Can you work these out from the model? Positions are in its coordinate system, mm. Face numbers are marked on the shaded views. A direction names the side the tool comes from. Coordinates: 2 decimals unless noted, no trailing zeros. Order: outer loops, then holes, each group sorted by start corner. A loop starts at its lowest first (then second) coordinate and runs counter-clockwise, first axis right, second up. Notation, with made-up numbers: (-26, -18.75) -> (11, -18.75) arc R12 ccw to (11, -4.75) -> close; hole circle Ø11 at (75.5, 80.25). An arc over 180 degrees is marked (long way). Answer in a Markdown table with one row per item.
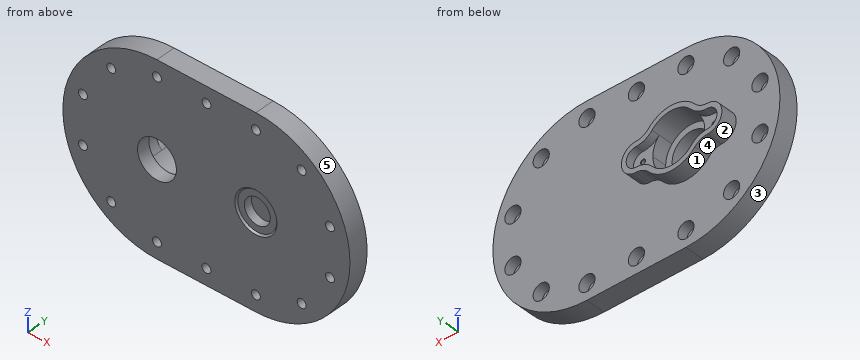
```python
from build123d import *

# Parameters (mm, degrees)
SKETCH2_R                   = 5
BOSS_EXTRUDE4_DEPTH         = 12
SKETCH2_6_R                 = 16
SKETCH2_6_R_2               = 12
BOSS_EXTRUDE5_DEPTH         = 8
SKETCH2_7_R                 = 1.25
BOSS_EXTRUDE6_DEPTH         = 17
BOSS_EXTRUDE7_DEPTH         = 22
SKETCH2_10_R                = 1.25
BOSS_EXTRUDE9_DEPTH         = 17
M3_TAPPED_HOLE2_D           = 2.5
M3_TAPPED_HOLE2_DEPTH       = 10
M3_TAPPED_HOLE2_CSINK_D     = 3.05
M3_TAPPED_HOLE2_CSINK_ANGLE = 90
M3_TAPPED_HOLE2_TIP         = 0.751075774
SKETCH11_R                  = 12
CUT_EXTRUDE1_DEPTH          = 1
SKETCH12_R                  = 8
CUT_EXTRUDE2_DEPTH          = 6
CHAMFER1_SIZE               = 1
SKETCH2_12_R                = 5
SKETCH2_12_R_2              = 2.75
BOSS_EXTRUDE10_DEPTH        = 5.8


with BuildPart() as part:
    # Sketch2 → Boss-Extrude4 (new body)
    with BuildSketch(Plane(origin=(0, 0, 0), x_dir=(1, 0, 0), z_dir=(0, 1, 0))):
        with BuildLine():
            Line((-61, -58), (0, -58))
            ThreePointArc((0, -58), (58, 0), (0, 58))
            Line((0, 58), (-61, 58))
            ThreePointArc((-61, 58), (-119, 0), (-61, -58))
        make_face()
        with Locations(Location((0, 48, 0), (0, 0, 270))):
            Circle(SKETCH2_R, mode=Mode.SUBTRACT)
        with Locations(Location((-30.5, 48, 0), (0, 0, 270))):
            Circle(SKETCH2_R, mode=Mode.SUBTRACT)
        with Locations(Location((-61, 48, 0), (0, 0, 270))):
            Circle(SKETCH2_R, mode=Mode.SUBTRACT)
        with Locations(Location((-89.21369211, 38.83281573, 0), (0, 0, 270))):
            Circle(SKETCH2_R, mode=Mode.SUBTRACT)
        with Locations(Location((-106.650712782, 14.83281573, 0), (0, 0, 270))):
            Circle(SKETCH2_R, mode=Mode.SUBTRACT)
        with Locations(Location((-106.650712782, -14.83281573, 0), (0, 0, 270))):
            Circle(SKETCH2_R, mode=Mode.SUBTRACT)
        with Locations(Location((-89.21369211, -38.83281573, 0), (0, 0, 270))):
            Circle(SKETCH2_R, mode=Mode.SUBTRACT)
        with Locations(Location((-61, -48, 0), (0, 0, 270))):
            Circle(SKETCH2_R, mode=Mode.SUBTRACT)
        with Locations(Location((-30.5, -48, 0), (0, 0, 270))):
            Circle(SKETCH2_R, mode=Mode.SUBTRACT)
        with Locations(Location((0, -48, 0), (0, 0, 270))):
            Circle(SKETCH2_R, mode=Mode.SUBTRACT)
        with Locations(Location((28.21369211, -38.83281573, 0), (0, 0, 270))):
            Circle(SKETCH2_R, mode=Mode.SUBTRACT)
        with Locations(Location((45.650712782, -14.83281573, 0), (0, 0, 270))):
            Circle(SKETCH2_R, mode=Mode.SUBTRACT)
        with Locations(Location((45.650712782, 14.83281573, 0), (0, 0, 270))):
            Circle(SKETCH2_R, mode=Mode.SUBTRACT)
        with Locations(Location((28.21369211, 38.83281573, 0), (0, 0, 270))):
            Circle(SKETCH2_R, mode=Mode.SUBTRACT)
        with BuildLine():
            ThreePointArc((-75.315068493, -12.493150685), (-61, -19), (-46.684931507, -12.493150685))
            ThreePointArc((-46.684931507, -12.493150685), (-43.220790032, -9.91426193), (-39, -9))
            ThreePointArc((-39, -9), (-30, 0), (-39, 9))
            ThreePointArc((-39, 9), (-43.220790032, 9.91426193), (-46.684931507, 12.493150685))
            ThreePointArc((-46.684931507, 12.493150685), (-61, 19), (-75.315068493, 12.493150685))
            ThreePointArc((-75.315068493, 12.493150685), (-78.779209968, 9.91426193), (-83, 9))
            ThreePointArc((-83, 9), (-92, 0), (-83, -9))
            ThreePointArc((-83, -9), (-78.779209968, -9.91426193), (-75.315068493, -12.493150685))
        make_face(mode=Mode.SUBTRACT)
    extrude(amount=BOSS_EXTRUDE4_DEPTH)



with BuildPart() as body_2:
    # Sketch2<6> → Boss-Extrude5 (new body)
    with BuildSketch(Plane(origin=(0, 0, 0), x_dir=(1, 0, 0), z_dir=(0, 1, 0))):
        with Locations(Location((-61, 0, 0), (0, 0, 270))):
            Circle(SKETCH2_6_R)
        with Locations(Location((-61, 0, 0), (0, 0, 270))):
            Circle(SKETCH2_6_R_2, mode=Mode.SUBTRACT)
    extrude(amount=BOSS_EXTRUDE5_DEPTH)

    # Sketch2<7> → Boss-Extrude6 (add)
    # profile 1 of 2: a face of its own
    with BuildSketch(Plane(origin=(0, 0, 0), x_dir=(1, 0, 0), z_dir=(0, 1, 0))):
        with BuildLine():
            ThreePointArc((-48.945205479, 10.520547945), (-46.018733159, 5.617975065), (-45, 0))
            ThreePointArc((-45, 0), (-46.018733159, -5.617975065), (-48.945205479, -10.520547945))
            ThreePointArc((-48.945205479, -10.520547945), (-44.462198865, -7.183162497), (-39, -6))
            ThreePointArc((-39, -6), (-33, 0), (-39, 6))
            ThreePointArc((-39, 6), (-44.462198865, 7.183162497), (-48.945205479, 10.520547945))
        make_face()
        with Locations(Location((-39, 0, 0), (0, 0, 270))):
            Circle(SKETCH2_7_R, mode=Mode.SUBTRACT)
    # profile 2 of 2: a face of its own
    with BuildSketch(Plane(origin=(0, 0, 0), x_dir=(1, 0, 0), z_dir=(0, 1, 0))):
        with BuildLine():
            ThreePointArc((-73.054794521, -10.520547945), (-77, 0), (-73.054794521, 10.520547945))
            ThreePointArc((-73.054794521, 10.520547945), (-77.537801135, 7.183162497), (-83, 6))
            ThreePointArc((-83, 6), (-89, 0), (-83, -6))
            ThreePointArc((-83, -6), (-77.537801135, -7.183162497), (-73.054794521, -10.520547945))
        make_face()
        with Locations(Location((-83, 0, 0), (0, 0, 270))):
            Circle(SKETCH2_7_R, mode=Mode.SUBTRACT)
    extrude(amount=BOSS_EXTRUDE6_DEPTH)


with BuildPart() as part_1:
    add(part.part)

    add(body_2.part)  # Boss-Extrude7 merges body 2
    # Sketch2<8> → Boss-Extrude7 (add)
    with BuildSketch(Plane(origin=(0, 0, 0), x_dir=(1, 0, 0), z_dir=(0, 1, 0))):
        with BuildLine():
            ThreePointArc((-46.684931507, -12.493150685), (-43.220790032, -9.91426193), (-39, -9))
            ThreePointArc((-39, -9), (-30, 0), (-39, 9))
            ThreePointArc((-39, 9), (-43.220790032, 9.91426193), (-46.684931507, 12.493150685))
            ThreePointArc((-46.684931507, 12.493150685), (-61, 19), (-75.315068493, 12.493150685))
            ThreePointArc((-75.315068493, 12.493150685), (-78.779209968, 9.91426193), (-83, 9))
            ThreePointArc((-83, 9), (-92, 0), (-83, -9))
            ThreePointArc((-83, -9), (-78.779209968, -9.91426193), (-75.315068493, -12.493150685))
            ThreePointArc((-75.315068493, -12.493150685), (-61, -19), (-46.684931507, -12.493150685))
        make_face()
        with BuildLine():
            ThreePointArc((-48.945205479, 10.520547945), (-44.462198865, 7.183162497), (-39, 6))
            ThreePointArc((-39, 6), (-33, 0), (-39, -6))
            ThreePointArc((-39, -6), (-44.462198865, -7.183162497), (-48.945205479, -10.520547945))
            ThreePointArc((-48.945205479, -10.520547945), (-61, -16), (-73.054794521, -10.520547945))
            ThreePointArc((-73.054794521, -10.520547945), (-77.537801135, -7.183162497), (-83, -6))
            ThreePointArc((-83, -6), (-89, 0), (-83, 6))
            ThreePointArc((-83, 6), (-77.537801135, 7.183162497), (-73.054794521, 10.520547945))
            ThreePointArc((-73.054794521, 10.520547945), (-61, 16), (-48.945205479, 10.520547945))
        make_face(mode=Mode.SUBTRACT)
    extrude(amount=BOSS_EXTRUDE7_DEPTH)

    # Sketch2<10> → Boss-Extrude9 (add)
    with BuildSketch(Plane(origin=(0, 0, 0), x_dir=(1, 0, 0), z_dir=(0, 1, 0))):
        with Locations((-39, 0)):
            Circle(SKETCH2_10_R)
        with Locations((-83, 0)):
            Circle(SKETCH2_10_R)
    extrude(amount=BOSS_EXTRUDE9_DEPTH)

    # M3 Tapped Hole2
    with Locations(Plane(origin=(0, 17, 0), x_dir=(1, 0, 0), z_dir=(0, 1, 0))):
        with Locations((-39, 0), (-83, 0)):
            CounterSinkHole(M3_TAPPED_HOLE2_D / 2, M3_TAPPED_HOLE2_CSINK_D / 2, depth=M3_TAPPED_HOLE2_DEPTH, counter_sink_angle=M3_TAPPED_HOLE2_CSINK_ANGLE)
            with Locations((0, 0, -(M3_TAPPED_HOLE2_DEPTH + M3_TAPPED_HOLE2_TIP / 2))):  # 118° drill point
                Cone(0, M3_TAPPED_HOLE2_D / 2, M3_TAPPED_HOLE2_TIP, mode=Mode.SUBTRACT)

    # Sketch11 → Cut-Extrude1 (cut)
    with BuildSketch(Plane.XZ):
        with Locations(Location((0, 0, 0), (0, 0, 270))):
            Circle(SKETCH11_R)
    extrude(amount=-CUT_EXTRUDE1_DEPTH, mode=Mode.SUBTRACT)

    # Sketch12 → Cut-Extrude2 (cut)
    with BuildSketch(Plane.XZ):
        with Locations(Location((0, 0, 0), (0, 0, 270))):
            Circle(SKETCH12_R)
    extrude(amount=-CUT_EXTRUDE2_DEPTH, mode=Mode.SUBTRACT)

    # Chamfer1
    chamfer1_edges = [part_1.edges().sort_by_distance(p)[0] for p in [
        (0, 0, 12),
    ]]
    chamfer(chamfer1_edges, length=CHAMFER1_SIZE - 0.0001)  # a hair under: the kernel refuses the full size

    # Sketch2<12> → Boss-Extrude10 (add)
    # profile 1 of 14: a face of its own
    with BuildSketch(Plane(origin=(0, 0, 0), x_dir=(1, 0, 0), z_dir=(0, 1, 0))):
        with Locations(Location((0, -48, 0), (0, 0, 270))):
            Circle(SKETCH2_12_R)
        with Locations(Location((0, -48, 0), (0, 0, 270))):
            Circle(SKETCH2_12_R_2, mode=Mode.SUBTRACT)
    # profile 2 of 14: a face of its own
    with BuildSketch(Plane(origin=(0, 0, 0), x_dir=(1, 0, 0), z_dir=(0, 1, 0))):
        with Locations(Location((28.21369211, -38.83281573, 0), (0, 0, 270))):
            Circle(SKETCH2_12_R)
        with Locations(Location((28.21369211, -38.83281573, 0), (0, 0, 270))):
            Circle(SKETCH2_12_R_2, mode=Mode.SUBTRACT)
    # profile 3 of 14: a face of its own
    with BuildSketch(Plane(origin=(0, 0, 0), x_dir=(1, 0, 0), z_dir=(0, 1, 0))):
        with Locations(Location((45.650712782, -14.83281573, 0), (0, 0, 270))):
            Circle(SKETCH2_12_R)
        with Locations(Location((45.650712782, -14.83281573, 0), (0, 0, 270))):
            Circle(SKETCH2_12_R_2, mode=Mode.SUBTRACT)
    # profile 4 of 14: a face of its own
    with BuildSketch(Plane(origin=(0, 0, 0), x_dir=(1, 0, 0), z_dir=(0, 1, 0))):
        with Locations(Location((45.650712782, 14.83281573, 0), (0, 0, 270))):
            Circle(SKETCH2_12_R)
        with Locations(Location((45.650712782, 14.83281573, 0), (0, 0, 270))):
            Circle(SKETCH2_12_R_2, mode=Mode.SUBTRACT)
    # profile 5 of 14: a face of its own
    with BuildSketch(Plane(origin=(0, 0, 0), x_dir=(1, 0, 0), z_dir=(0, 1, 0))):
        with Locations(Location((28.21369211, 38.83281573, 0), (0, 0, 270))):
            Circle(SKETCH2_12_R)
        with Locations(Location((28.21369211, 38.83281573, 0), (0, 0, 270))):
            Circle(SKETCH2_12_R_2, mode=Mode.SUBTRACT)
    # profile 6 of 14: a face of its own
    with BuildSketch(Plane(origin=(0, 0, 0), x_dir=(1, 0, 0), z_dir=(0, 1, 0))):
        with Locations(Location((0, 48, 0), (0, 0, 270))):
            Circle(SKETCH2_12_R)
        with Locations(Location((0, 48, 0), (0, 0, 270))):
            Circle(SKETCH2_12_R_2, mode=Mode.SUBTRACT)
    # profile 7 of 14: a face of its own
    with BuildSketch(Plane(origin=(0, 0, 0), x_dir=(1, 0, 0), z_dir=(0, 1, 0))):
        with Locations(Location((-30.5, 48, 0), (0, 0, 270))):
            Circle(SKETCH2_12_R)
        with Locations(Location((-30.5, 48, 0), (0, 0, 270))):
            Circle(SKETCH2_12_R_2, mode=Mode.SUBTRACT)
    # profile 8 of 14: a face of its own
    with BuildSketch(Plane(origin=(0, 0, 0), x_dir=(1, 0, 0), z_dir=(0, 1, 0))):
        with Locations(Location((-61, 48, 0), (0, 0, 270))):
            Circle(SKETCH2_12_R)
        with Locations(Location((-61, 48, 0), (0, 0, 270))):
            Circle(SKETCH2_12_R_2, mode=Mode.SUBTRACT)
    # profile 9 of 14: a face of its own
    with BuildSketch(Plane(origin=(0, 0, 0), x_dir=(1, 0, 0), z_dir=(0, 1, 0))):
        with Locations(Location((-89.21369211, 38.83281573, 0), (0, 0, 270))):
            Circle(SKETCH2_12_R)
        with Locations(Location((-89.21369211, 38.83281573, 0), (0, 0, 270))):
            Circle(SKETCH2_12_R_2, mode=Mode.SUBTRACT)
    # profile 10 of 14: a face of its own
    with BuildSketch(Plane(origin=(0, 0, 0), x_dir=(1, 0, 0), z_dir=(0, 1, 0))):
        with Locations(Location((-106.650712782, 14.83281573, 0), (0, 0, 270))):
            Circle(SKETCH2_12_R)
        with Locations(Location((-106.650712782, 14.83281573, 0), (0, 0, 270))):
            Circle(SKETCH2_12_R_2, mode=Mode.SUBTRACT)
    # profile 11 of 14: a face of its own
    with BuildSketch(Plane(origin=(0, 0, 0), x_dir=(1, 0, 0), z_dir=(0, 1, 0))):
        with Locations(Location((-106.650712782, -14.83281573, 0), (0, 0, 270))):
            Circle(SKETCH2_12_R)
        with Locations(Location((-106.650712782, -14.83281573, 0), (0, 0, 270))):
            Circle(SKETCH2_12_R_2, mode=Mode.SUBTRACT)
    # profile 12 of 14: a face of its own
    with BuildSketch(Plane(origin=(0, 0, 0), x_dir=(1, 0, 0), z_dir=(0, 1, 0))):
        with Locations(Location((-89.21369211, -38.83281573, 0), (0, 0, 270))):
            Circle(SKETCH2_12_R)
        with Locations(Location((-89.21369211, -38.83281573, 0), (0, 0, 270))):
            Circle(SKETCH2_12_R_2, mode=Mode.SUBTRACT)
    # profile 13 of 14: a face of its own
    with BuildSketch(Plane(origin=(0, 0, 0), x_dir=(1, 0, 0), z_dir=(0, 1, 0))):
        with Locations(Location((-61, -48, 0), (0, 0, 270))):
            Circle(SKETCH2_12_R)
        with Locations(Location((-61, -48, 0), (0, 0, 270))):
            Circle(SKETCH2_12_R_2, mode=Mode.SUBTRACT)
    # profile 14 of 14: a face of its own
    with BuildSketch(Plane(origin=(0, 0, 0), x_dir=(1, 0, 0), z_dir=(0, 1, 0))):
        with Locations(Location((-30.5, -48, 0), (0, 0, 270))):
            Circle(SKETCH2_12_R)
        with Locations(Location((-30.5, -48, 0), (0, 0, 270))):
            Circle(SKETCH2_12_R_2, mode=Mode.SUBTRACT)
    extrude(amount=BOSS_EXTRUDE10_DEPTH)


solid = part_1.part
```
(1) Suppose I cut it at C-C (z = -48). Please give me the cut outline in (x, y).
Response values:
| item | result |
|---|---|
| outline | (-93.56, 0) -> (-63.75, 0) -> (-63.75, 5.8) -> (-66, 5.8) -> (-66, 12) -> (-93.56, 12) -> close; (-58.25, 0) -> (-33.25, 0) -> (-33.25, 5.8) -> (-35.5, 5.8) -> (-35.5, 12) -> (-56, 12) -> (-56, 5.8) -> (-58.25, 5.8) -> close; (-27.75, 0) -> (-2.75, 0) -> (-2.75, 5.8) -> (-5, 5.8) -> (-5, 12) -> (-25.5, 12) -> (-25.5, 5.8) -> (-27.75, 5.8) -> close; (2.75, 0) -> (32.56, 0) -> (32.56, 12) -> (5, 12) -> (5, 5.8) -> (2.75, 5.8) -> close |
(2) Suppose I cut it at B-B (x = -52). Please give me the cut outline in (y, z).
Response values:
| item | result |
|---|---|
| outline | (0, -58) -> (12, -58) -> (12, -16.73) -> (22, -16.73) -> (22, -13.23) -> (8, -13.23) -> (8, -7.94) -> (0, -7.94) -> close; (0, 7.94) -> (8, 7.94) -> (8, 13.23) -> (22, 13.23) -> (22, 16.73) -> (12, 16.73) -> (12, 58) -> (0, 58) -> close |
(3) Suppose I cut it at D-D (y = 3.25). Count the separate pieces of the cut face and the enclosed holes in it, and give its area (3 significant figures).
Response values:
| item | result |
|---|---|
| separate pieces | 1 |
| enclosed holes | 16 |
| area | 16,700 mm2 |
(4) On a 3-axis mill with a long thin cutter (end or side, diameter ignored), from which of +Z, -Z, +X, -X, +Y, -Y can I reach the whole of each face in a straight line? I mean the marked faces 1, 2, 3, 4 and 5. Say none if no direction works.
Response values:
| item | result |
|---|---|
| face 1 | -Z, +Y |
| face 2 | -X, +Y |
| face 3 | -X, +Y, -Y |
| face 4 | -Z, -X, +Y |
| face 5 | +X, +Y, -Y |
(5) Will these pins go through, and if not, where does the flat tip stop? pin 1 Ø3 at (x, z) = (-49.5, 42.5) entering from +Y; pin 2 Ø8 at (x, z) = (-42.5, -4.5) entering from +Y; pin 3 Ø5 at (y, z) = (12, 28.5) entering from +X; pin 4 Ø3 at (x, y) = (-66, 19.5) entering from +Z.
Response values:
| item | result |
|---|---|
| pin 1 | y = 12 |
| pin 2 | y = 22 |
| pin 3 | x = 51.85 |
| pin 4 | z = 18.67 |
(6) Suppose I cut it at A-A (y = 20). Please give me the cut outline in (x, z), and give its area (3 significant figures).
Response values:
| item | result |
|---|---|
| outline | (-83, -9) arc R10.2 cw to (-75.32, -12.49) arc R19 ccw to (-46.68, -12.49) arc R10.2 cw to (-39, -9) arc R9 ccw to (-39, 9) arc R10.2 cw to (-46.68, 12.49) arc R19 ccw to (-75.32, 12.49) arc R10.2 cw to (-83, 9) arc R9 ccw to start; hole (-83, -6) arc R13.2 cw to (-73.05, -10.52) arc R16 ccw to (-48.95, -10.52) arc R13.2 cw to (-39, -6) arc R6 ccw to (-39, 6) arc R13.2 cw to (-48.95, 10.52) arc R16 ccw to (-73.05, 10.52) arc R13.2 cw to (-83, 6) arc R6 ccw to start |
| area | 440 mm2 |
(7) I need wall thicknesses on line 1 (Z direction, x = 45, y = 9.5); line 2 (X direction, y = 6.5, z = -46); line 3 (Y direction, x = -42, z = 52). Which ranges of each line are inside material? Lowest first, please. Write a range as [from, to].
Response values:
| item | result |
|---|---|
| line 1 | [-36.59, -19.79], [-9.88, 9.88], [19.79, 36.59] |
| line 2 | [-96.33, -65.58], [-56.42, -35.08], [-25.92, -4.58], [4.58, 35.33] |
| line 3 | [0, 12] |
